Job drawing, mm, ordinate dimensions from the low corner. One solid piece. A direction names the side the tool comes from. Give positions to 0.01 mm unless a question says otherwise; leave off trailing zeros. Loops run counter-clockwise (first coordinate to the right, second up) from the corner with the lowest first, then second, coordinate; pieces in that order, holes last. Notation, with made-up numbers: M 39,74.25 L 92,74.25 A18 cw 92,88.25 Z; hole C -29,-8 d6. An arc over 180 degrees is marked long. Put each result on its own line as item: value.
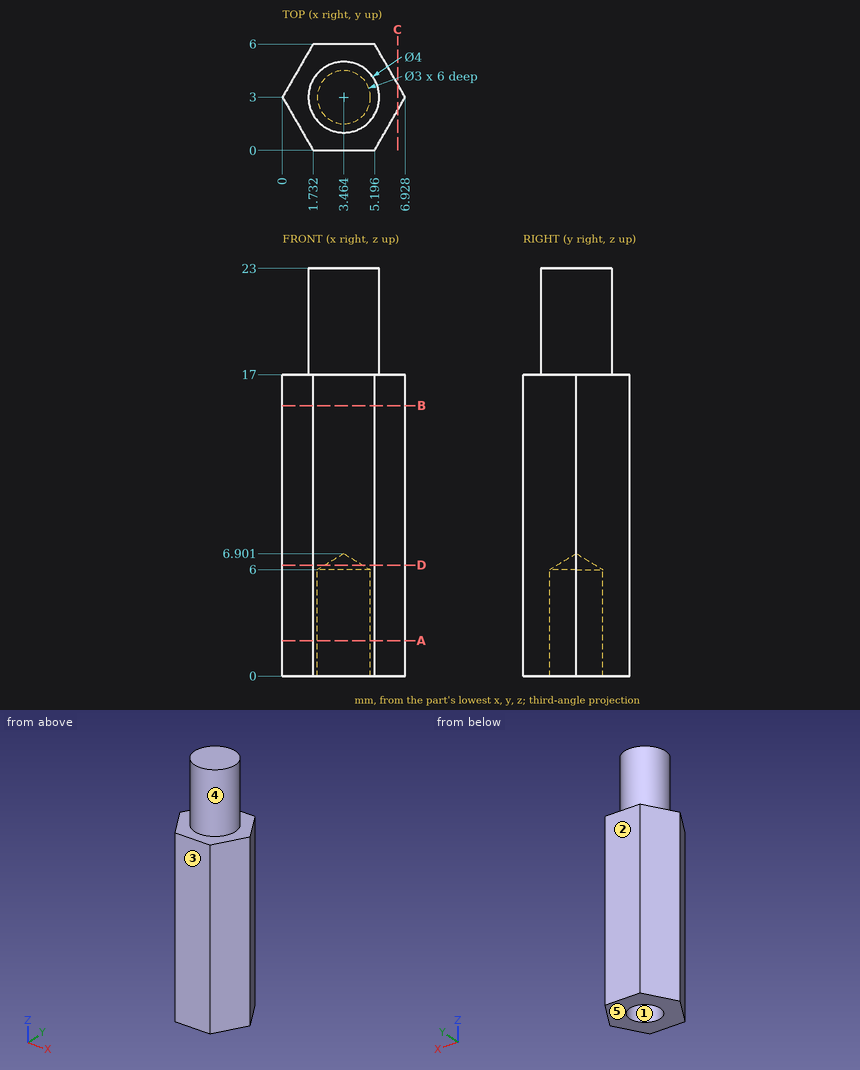
Q1. Slice it at A-A (z = 2). List the corners of the cut face in (x, y).
Here are the results:
outline: M 0,3 L 1.73,0 L 5.2,0 L 6.93,3 L 5.2,6 L 1.73,6 Z; hole C 3.46,3 d3
Q2. Slice it at D-D (z = 6.25). List the corners of the cut face in (x, y).
Here are the results:
outline: M 0,3 L 1.73,0 L 5.2,0 L 6.93,3 L 5.2,6 L 1.73,6 Z; hole C 3.46,3 d2.17
Q3. Drop a flat-ended pin along its axis: pin 1 Ø1.5 at (x, z) = (3.5, 19.5) entering from -Y. Give the stop position or say it passes through.
Here are the results:
pin 1: y = 1
Q4. Mould opens along Y. For the marked faces 1, 2 and 3 say: pulls with the +Y half, pulls with the -Y half, needs draft (parallel to the pull), parting line crosses it, or undercut.
Here are the results:
face 1: undercut
face 2: pulls with the +Y half
face 3: pulls with the -Y half
Q5. Probe line 1 (Z direction, x = 1.75, y = 4.25); line 2 (Y direction, x = 3.25, z = 2) (1 decimal); line 3 (Y direction, x = 2.5, z = 3). List the from-to ranges inside material, lowest first. Write a range as from..to.
Here are the results:
line 1: 0..17
line 2: 0..1.5, 4.5..6
line 3: 0..1.85, 4.15..6
Q6. Slice it at B-B (z = 15.25). List the corners of the cut face in (x, y).
Here are the results:
outline: M 0,3 L 1.73,0 L 5.2,0 L 6.93,3 L 5.2,6 L 1.73,6 Z
Q7. Slice it at C-C (x = 6.5). List the corners of the cut face in (y, z), and give its area (3 significant figures).
Here are the results:
outline: M 2.26,0 L 3.74,0 L 3.74,17 L 2.26,17 Z
area: 25.2 mm²
Q8. Tool access for the marked faces 4 and 5: list every direction of +Z, -Z, +X, -X, +Y, -Y with a clear straight run to the whole face (end or side of a thin tool).
Here are the results:
face 4: +Z
face 5: -Z, +X, -X, +Y, -Y
